from build123d import *

# Parameters (mm, degrees)
SKETCH_1_R          = 2.75
EXTRUDE_1_DEPTH     = 4
SKETCH_2_R          = 2.75
EXTRUDE_2_DEPTH     = 4
FILLET_2_R          = 4
FILLET_3_R          = 8
FILLET_4_R          = 25
CUT_EXTRUDE_1_DEPTH = 5


with BuildPart() as part:
    # Эскиз1 → Бобышка-Вытянуть1 (new body)
    with BuildSketch(Plane.XY):
        Polygon((18, 0), (-18, 0), (-18, 23), (-30, 23), (-30, -7), (-40, -7), (-40, -32), (40, -32), (40, -7), (30, -7), (30, 23), (18, 23), align=None)
        with Locations((-23, 18)):
            Circle(SKETCH_1_R, mode=Mode.SUBTRACT)
        with Locations((-23, 0)):
            Circle(SKETCH_1_R, mode=Mode.SUBTRACT)
        with Locations((-33, -26)):
            Circle(SKETCH_1_R, mode=Mode.SUBTRACT)
        with Locations((0, -26)):
            Circle(SKETCH_1_R, mode=Mode.SUBTRACT)
        with Locations((33, -26)):
            Circle(SKETCH_1_R, mode=Mode.SUBTRACT)
        with Locations((23, 18)):
            Circle(SKETCH_1_R, mode=Mode.SUBTRACT)
        with Locations((23, 0)):
            Circle(SKETCH_1_R, mode=Mode.SUBTRACT)
    extrude(amount=EXTRUDE_1_DEPTH)

    # Эскиз2 → Бобышка-Вытянуть2 (add)
    with BuildSketch(Plane.XY):
        Polygon((17.5, 0), (-17.5, 0), (-17.5, 23), (-30, 23), (-40, -7), (-40, -32), (-40, -48), (40, -48), (40, -32), (40, -7), (30, 23), (17.5, 23), align=None)
        with Locations((-23, 18)):
            Circle(SKETCH_2_R, mode=Mode.SUBTRACT)
        with Locations((-23, 0)):
            Circle(SKETCH_2_R, mode=Mode.SUBTRACT)
        with Locations((-33, -26)):
            Circle(SKETCH_2_R, mode=Mode.SUBTRACT)
        with Locations((-33, -42)):
            Circle(SKETCH_2_R, mode=Mode.SUBTRACT)
        with Locations((33, -26)):
            Circle(SKETCH_2_R, mode=Mode.SUBTRACT)
        with Locations((23, 18)):
            Circle(SKETCH_2_R, mode=Mode.SUBTRACT)
        with Locations((23, 0)):
            Circle(SKETCH_2_R, mode=Mode.SUBTRACT)
        with Locations((33, -42)):
            Circle(SKETCH_2_R, mode=Mode.SUBTRACT)
    extrude(amount=EXTRUDE_2_DEPTH)

    # Скругление2
    fillet_2_edges = [part.edges().sort_by_distance(p)[0] for p in [
        (-17.5, 23, 2),
        (40, -48, 2),
        (-40, -48, 2),
        (17.5, 23, 2),
    ]]
    fillet(fillet_2_edges, radius=FILLET_2_R)

    # Скругление3
    fillet_3_edges = [part.edges().sort_by_distance(p)[0] for p in [
        (30, 23, 2),
        (-30, 23, 2),
    ]]
    fillet(fillet_3_edges, radius=FILLET_3_R)

    # Скругление4
    fillet_4_edges = [part.edges().sort_by_distance(p)[0] for p in [
        (40, -7, 2),
        (-40, -7, 2),
    ]]
    fillet(fillet_4_edges, radius=FILLET_4_R)

    # Эскиз3 → Вырез-Вытянуть1 (cut, through all)
    with BuildSketch(Plane.XY.offset(4)):
        with BuildLine():
            Line((-12.5, -18.5), (12.5, -18.5))
            ThreePointArc((12.5, -18.5), (25, -31), (12.5, -43.5))
            Line((12.5, -43.5), (-12.5, -43.5))
            ThreePointArc((-12.5, -43.5), (-25, -31), (-12.5, -18.5))
        make_face()
    extrude(amount=-CUT_EXTRUDE_1_DEPTH, mode=Mode.SUBTRACT)


solid = part.part
Could you check a few things on this model? Use its own coordinates, in mm. A direction names the side the tool comes from. Coordinates: 2 decimals unless noted, no trailing zeros. Order: outer loops, then holes, each group sorted by start corner. A loop starts at its lowest first (then second) coordinate and runs counter-clockwise, first axis right, second up. Notation, with made-up numbers: (47, 48.25) -> (82, 48.25) arc R34 cw to (82, 81.25) -> close; hole circle Ø3 at (9, -10). An arc over 180 degrees is marked (long way). One line per item, written item: value. Start each with the question number.
1) We'd pull the mould along X, two halves only. Please class faces 1 (the flat face through (0, -18.5, 2)), 2 (the flat face through (-35.222, 7.334, 1.972)), 3 (the cylindrical face through (-25.747, 18.121, 1.972)), 4 (the cylindrical face through (39.686, -7.108, 2.028)): +X half, -X half, draft (parallel to the pull), parting line (faces both ways), or undercut.
2) Imagine slicing it at C-C on z = 1.8. Count the separate pieces of the cut face and the enclosed holes in it, plus the area to 3 significant figures.
3) Imagine slicing it at B-B on x = -4. List the corners of the cut face in (y, z) for me.
4) Which directions (+Z, -Z, +X, -X, +Y, -Y) give clear straight access to the entire face, cutting with the end or side of a thin tool? Please do faces 5 (the cylindrical face through (18.703, 21.859, 2.028)), 6 (the cylindrical face through (25, -31, 2)), 7 (the flat face through (-23, 23, 2)).
5) Imagine slicing it at A-A on y = -31. List the corners of the cut face in (x, z) for me.
6) I'm going to push flat-ended pins straight in: pin 1 (1.2 mm diameter, centred on y = 14, z = 2.5, fed in from +X); pin 2 (1 mm diameter, centred on y = 12.5, z = 2.5, fed in from -X). Where does each tip first touch, or does it pass through?
7) If I drill on L1, parallel to Y at x = -5, z = 1.4; L2, parallel to Y at x = -23, z = 1.25; L3, parallel to X at y = -41, z = 3.35, over which ranges is the centre line in solid material (lowest first)? Write a range as [from, to].
8) Imagine slicing it at D-D on x = -33. List the corners of the cut face in (y, z) for me.
Answer list:
1. face 1: undercut
1. face 2: -X half
1. face 3: undercut
1. face 4: +X half
2. separate pieces: 1
2. enclosed holes: 9
2. area: 3,240 mm2
3. outline: (-48, 0) -> (-43.5, 0) -> (-43.5, 4) -> (-48, 4) -> close; (-18.5, 0) -> (0, 0) -> (0, 4) -> (-18.5, 4) -> close
4. face 5: +Z, -Z, +Y
4. face 6: +Z, -Z
4. face 7: +Z, -Z, +X, -X, +Y
5. outline: (-40, 0) -> (-25, 0) -> (-25, 4) -> (-40, 4) -> close; (25, 0) -> (40, 0) -> (40, 4) -> (25, 4) -> close
6. pin 1: stops at x = 33.2
6. pin 2: stops at x = -33.67
7. L1: y = [-48, -43.5], [-18.5, 0]
7. L2: y = [-48, -37.78], [-24.22, -2.75], [2.75, 15.25], [20.75, 23]
7. L3: x = [-40, -35.56], [-30.44, -20], [20, 30.44], [35.56, 40]
8. outline: (-48, 0) -> (-44.75, 0) -> (-44.75, 4) -> (-48, 4) -> close; (-39.25, 0) -> (-28.75, 0) -> (-28.75, 4) -> (-39.25, 4) -> close; (-23.25, 0) -> (14, 0) -> (14, 4) -> (-23.25, 4) -> close
